```python
from build123d import *

# Parameters (mm, degrees)
SKETCH1_W           = 16.1
SKETCH1_H           = 16.1
SKETCH1_W_2         = 14.1
SKETCH1_H_2         = 14.1
BOSS_EXTRUDE1_DEPTH = 10
SKETCH1_2_W         = 14.1
SKETCH1_2_H         = 14.1
BOSS_EXTRUDE2_DEPTH = 4
SKETCH2_R           = 2.625
BOSS_EXTRUDE3_DEPTH = 6
CHAMFER1_SIZE       = 0.1
FILLET1_R           = 0.5


with BuildPart() as part:
    # Sketch1 → Boss-Extrude1 (new body)
    with BuildSketch(Plane(origin=(0, 0, 0), x_dir=(1, 0, 0), z_dir=(0, 1, 0))):
        Rectangle(SKETCH1_W, SKETCH1_H)
        Rectangle(SKETCH1_W_2, SKETCH1_H_2, mode=Mode.SUBTRACT)
    extrude(amount=BOSS_EXTRUDE1_DEPTH)

    # Sketch1<2> → Boss-Extrude2 (add)
    with BuildSketch(Plane(origin=(0, 0, 0), x_dir=(1, 0, 0), z_dir=(0, 1, 0))):
        Rectangle(SKETCH1_2_W, SKETCH1_2_H)
    extrude(amount=BOSS_EXTRUDE2_DEPTH)

    # Sketch2 → Boss-Extrude3 (add)
    with BuildSketch(Plane(origin=(0, 4, 0), x_dir=(1, 0, 0), z_dir=(0, 1, 0))):
        with Locations(Location((0, 0, 0), (0, 0, 90))):
            Circle(SKETCH2_R)
        with BuildLine():
            Line((-0.9, -0.6), (-2.075, -0.6))
            Line((-2.075, -0.6), (-2.075, 0.6))
            Line((-2.075, 0.6), (-0.9, 0.6))
            ThreePointArc((-0.9, 0.6), (-0.687867966, 0.687867966), (-0.6, 0.9))
            Line((-0.6, 0.9), (-0.6, 2.075))
            Line((-0.6, 2.075), (0.6, 2.075))
            Line((0.6, 2.075), (0.6, 0.9))
            ThreePointArc((0.6, 0.9), (0.687867966, 0.687867966), (0.9, 0.6))
            Line((0.9, 0.6), (2.075, 0.6))
            Line((2.075, 0.6), (2.075, -0.6))
            Line((2.075, -0.6), (0.9, -0.6))
            ThreePointArc((0.9, -0.6), (0.687867966, -0.687867966), (0.6, -0.9))
            Line((0.6, -0.9), (0.6, -2.075))
            Line((0.6, -2.075), (-0.6, -2.075))
            Line((-0.6, -2.075), (-0.6, -0.9))
            ThreePointArc((-0.6, -0.9), (-0.687867966, -0.687867966), (-0.9, -0.6))
        make_face(mode=Mode.SUBTRACT)
    extrude(amount=BOSS_EXTRUDE3_DEPTH)

    # Chamfer1
    chamfer1_edges = [part.edges().sort_by_distance(p)[0] for p in [
        (0.687867966, 10, 0.687867966),
        (0, 10, 2.075),
        (-0.6, 10, 1.4875),
        (-0.687867966, 10, 0.687867966),
        (-2.075, 10, 0),
        (-1.4875, 10, -0.6),
        (-0.687867966, 10, -0.687867966),
        (-0.6, 10, -1.4875),
        (0.687867966, 10, -0.687867966),
        (1.4875, 10, -0.6),
        (1.4875, 10, 0.6),
        (0.6, 10, 1.4875),
        (-1.4875, 10, 0.6),
        (0, 10, -2.075),
        (0.6, 10, -1.4875),
        (2.075, 10, 0),
    ]]
    chamfer(chamfer1_edges, length=CHAMFER1_SIZE)

    # Fillet1
    fillet1_edges = [part.edges().sort_by_distance(p)[0] for p in [
        (8.05, 5, 8.05),
        (-8.05, 5, 8.05),
        (-8.05, 5, -8.05),
        (8.05, 5, -8.05),
    ]]
    fillet(fillet1_edges, radius=FILLET1_R)


solid = part.part
```
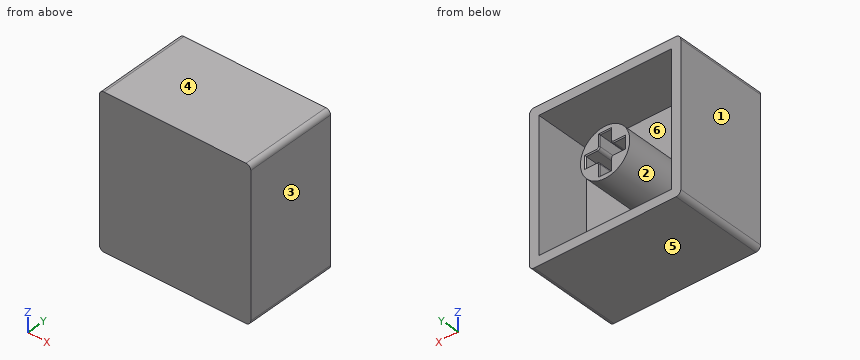
The listing builds one solid part. Answer for the finished solid, in the listing's coordinates (mm). Face numbers are marked on the shaded views. A direction names the side the tool comes from. Round coordinates to 2 decimals unless told otherwise and drop trailing zeros. Loops run counter-clockwise (first coordinate to the right, second up) from the corner with the lowest first, then second, coordinate; pieces in that order, holes last. Notation, with made-up numbers: (72, 0) -> (99, 0) arc R30 cw to (99, 23) -> close; hole circle Ø9 at (36, 12). An arc over 180 degrees is marked (long way). Use one line per item in the form item = value.
1. A flat-ended cylindrical pin translates along its axis: pin 1 Ø3 at (x, z) = (2.5, -4) entering from +Y. Find the tip coordinate at first contact, or state that the pin passes through.
Answer key:
pin_1 = 4
2. Find the intervals of material crossed by probe 1 along Z at (x, y) = (-5.25, 5); probe 2 along X at (y, z) = (9, 0) (3 decimals), in increasing order. Write a range as [from, to].
Answer key:
probe_1 = [-8.05, -7.05], [7.05, 8.05]
probe_2 = [-8.05, -7.05], [-2.625, -2.075], [2.075, 2.625], [7.05, 8.05]
3. The part is cut by section C-C on z = 0. Determine the outline of the cut face in (x, y) (3 decimals), and give its area (3 significant figures).
Answer key:
outline = (-8.05, 0) -> (8.05, 0) -> (8.05, 10) -> (7.05, 10) -> (7.05, 4) -> (2.625, 4) -> (2.625, 10) -> (2.175, 10) -> (2.075, 9.9) -> (2.075, 4) -> (-2.075, 4) -> (-2.075, 9.9) -> (-2.175, 10) -> (-2.625, 10) -> (-2.625, 4) -> (-7.05, 4) -> (-7.05, 10) -> (-8.05, 10) -> close
area = 83.0 mm²
4. The part is cut by section D-D on x = 3.25. Determine the outline of the cut face in (y, z), and give its area (3 significant figures).
Answer key:
outline = (0, -8.05) -> (10, -8.05) -> (10, -7.05) -> (4, -7.05) -> (4, 7.05) -> (10, 7.05) -> (10, 8.05) -> (0, 8.05) -> close
area = 76.4 mm²
5. A tool of negligible diameter and unlimited length cuts with its end or side. For the marked faces 1 and 2, from which of +Z, -Z, +X, -X, +Y, -Y can it reach the whole face along a straight path? Write none if from no direction.
Answer key:
face_1 = +Z, -Z, -X, +Y, -Y
face_2 = +Y
6. The part is cut by section A-A on y = 4.25. Give the number of separate pieces and of enclosed holes in the cut face, and give its area (3 significant figures).
Answer key:
separate_pieces = 2
enclosed_holes = 2
area = 73.2 mm²
7. The part is cut by section B-B on x = 0. Determine the outline of the cut face in (y, z) (3 decimals).
Answer key:
outline = (0, -8.05) -> (10, -8.05) -> (10, -7.05) -> (4, -7.05) -> (4, -2.625) -> (10, -2.625) -> (10, -2.175) -> (9.9, -2.075) -> (4, -2.075) -> (4, 2.075) -> (9.9, 2.075) -> (10, 2.175) -> (10, 2.625) -> (4, 2.625) -> (4, 7.05) -> (10, 7.05) -> (10, 8.05) -> (0, 8.05) -> close
8. For a pull along Z with two mould halves and no side action, classify the marked faces 3, 4, 5 and 6 as released by +Z, released by -Z, zero draft, split by the parting line, or undercut.
Answer key:
face_3 = zero draft
face_4 = released by +Z
face_5 = released by -Z
face_6 = undercut
